For this review, take the finished solid that the model builds, in its own axes (mm). A direction names the side the tool comes from. Round coordinates to 2 decimals unless told otherwise and drop trailing zeros. Write each loop counter-clockwise with the first axis right and the second up, starting at its lowest first coordinate (ties: lowest second). Pieces come first, ordered by that corner, then holes. Notation, with made-up numbers: M 15.5,34.5 L 42.5,34.5 A10 cw 42.5,40.5 Z; hole C -13.75,52 d11. An arc over 180 degrees is marked long. Use one line per item in the form item = value. Start each with the question number.
Item 1: Add section B-B (z = 43.5). State the section outline as (x, y) points.
Item 2: Add section A-A (y = -4.5). State the section outline as (x, z) points.
Item 3: Add section C-C (x = -16). State the section outline as (y, z) points, and give its area (3 significant figures).
Item 4: For faces 5 (the flat face through (0, 0, 1)), 6 (the flat face through (45, 8, 1)), 7 (the flat face through (-30, 7, 1)), list the 3-axis set-ups (+Z, -Z, +X, -X, +Y, -Y) from which the entire face can be reached by the end or side of a thin tool; tool diameter is ignored.
Item 5: Draft analysis for pull direction Y (two halves, no side actions). For faces 1 (the flat face through (54, -8, 1)), 2 (the flat face through (-58, 0, 1)), 3 (the flat face through (30, 7, 1)), 4 (the flat face through (-46, 11, -1)), state which applies: released by +Y, released by -Y, zero draft, split by the parting line, or undercut.
Item 6: For P1, Ø8, axis at x = 10.5, z = 25.5, coming from the +Y side; P2, Ø8, axis at x = 11.5, z = 0, coming from the -Y side; P3, Ø5, axis at x = -0.5, y = -1, coming from the +Z side; P4, Ø6, axis at x = -46.5, z = 70.5, coming from the -Y side, all flat-tipped, find the tip position at first contact; note any pin that passes through.
Item 7: For line 1 (X direction, y = 0.75, z = 71); line 2 (X direction, y = 7.75, z = -4); line 3 (Y direction, x = -56, z = -25), list the stretches that pass through material, from the lowest coordinate up. Write a range as [from, to].
from build123d import *

# Parameters (mm, degrees)
BOSS_EXTRUDE1_DEPTH      = 90
BOSS_EXTRUDE1_DEPTH_BACK = 90
SKETCH1_W                = 122
SKETCH1_H                = 22
SKETCH2_W                = 25
SKETCH2_H                = 16
CUT_EXTRUDE1_DEPTH       = 191.373317458
SKETCH3_W                = 60
SKETCH3_H                = 16
CUT_EXTRUDE2_DEPTH       = 191.373317458
SKETCH4_W                = 60.154663558
SKETCH4_H                = 22
CUT_EXTRUDE3_DEPTH       = 191.373317458
SKETCH5_W                = 20.922668221
SKETCH5_H                = 11
CUT_EXTRUDE4_DEPTH       = 191.373317458


with BuildPart() as part:
    # Sketch1 → Boss-Extrude1 (new, two sides: drawn at the far end of the back side and taken through both)
    with BuildSketch(Plane.XY.offset(-BOSS_EXTRUDE1_DEPTH_BACK)):
        Rectangle(SKETCH1_W, SKETCH1_H)
    extrude(amount=BOSS_EXTRUDE1_DEPTH + BOSS_EXTRUDE1_DEPTH_BACK)

    # Sketch2 → Cut-Extrude1 (cut, symmetric)
    with BuildSketch(Plane.XY.offset(90)):
        with Locations((45.5, 0)):
            Rectangle(SKETCH2_W, SKETCH2_H)
    cut_extrude1 = extrude(amount=CUT_EXTRUDE1_DEPTH, both=True, mode=Mode.SUBTRACT)

    # Mirror1: Cut-Extrude1 across plane
    add(cut_extrude1.mirror(Plane(origin=(0, 0, 0), x_dir=(0, 0, 1), z_dir=(1, 0, 0))), mode=Mode.SUBTRACT)

    # Sketch3 → Cut-Extrude2 (cut, through all)
    with BuildSketch(Plane.XY.offset(90)):
        with Locations((0, 11)):
            Rectangle(SKETCH3_W, SKETCH3_H)
    extrude(amount=-CUT_EXTRUDE2_DEPTH, mode=Mode.SUBTRACT)

    # Sketch4 → Cut-Extrude3 (cut, through all)
    with BuildSketch(Plane.XY.offset(90)):
        with Locations((0, -11)):
            Rectangle(SKETCH4_W, SKETCH4_H)
    extrude(amount=-CUT_EXTRUDE3_DEPTH, mode=Mode.SUBTRACT)

    # Sketch5 → Cut-Extrude4 (cut, through all)
    with BuildSketch(Plane.XY.offset(90)):
        with Locations((40.53866589, -5.5)):
            Rectangle(SKETCH5_W, SKETCH5_H)
    cut_extrude4 = extrude(amount=-CUT_EXTRUDE4_DEPTH, mode=Mode.SUBTRACT)

    # Mirror2: Cut-Extrude4 across plane
    add(cut_extrude4.mirror(Plane(origin=(0, 0, 0), x_dir=(0, 0, 1), z_dir=(1, 0, 0))), mode=Mode.SUBTRACT)


solid = part.part
Calculated:
q1.outline = M -61,-11 L -51,-11 L -51,-8 L -58,-8 L -58,8 L -33,8 L -33,0 L 33,0 L 33,8 L 58,8 L 58,-8 L 51,-8 L 51,-11 L 61,-11 L 61,11 L 30,11 L 30,3 L -30,3 L -30,11 L -61,11 Z
q2.outline = M -61,-90 L -58,-90 L -58,90 L -61,90 Z; M 58,-90 L 61,-90 L 61,90 L 58,90 Z
q3.outline = M 0,-90 L 3,-90 L 3,90 L 0,90 Z
q3.area = 540 mm^2
q4.face_5 = +Z, -Z, -Y
q4.face_6 = +Z, -Z
q4.face_7 = +Z, -Z, +Y
q5.face_1 = undercut
q5.face_2 = undercut
q5.face_3 = zero draft
q5.face_4 = released by +Y
q6.P1 = 3
q6.P2 = 0
q6.P3 = 90
q6.P4 = 8
q7.line_1 = [-61, -58], [-33, 33], [58, 61]
q7.line_2 = [-61, -58], [-33, -30], [30, 33], [58, 61]
q7.line_3 = [-11, -8], [8, 11]
